```python
from build123d import *

# Parameters (mm, degrees)
SKETCH1_R           = 35.8013
SKETCH1_R_2         = 32.754
BOSS_EXTRUDE1_DEPTH = 15.875
CHAMFER1_SIZE       = 1.27


with BuildPart() as part:
    # Sketch1 → Boss-Extrude1 (new body, symmetric)
    with BuildSketch(Plane.XY):
        Circle(SKETCH1_R)
        Circle(SKETCH1_R_2, mode=Mode.SUBTRACT)
    extrude(amount=BOSS_EXTRUDE1_DEPTH, both=True)

    # Chamfer1
    chamfer1_edges = [part.edges().sort_by_distance(p)[0] for p in [
        (-32.754, 0, -15.875),
        (-32.754, 0, 15.875),
    ]]
    chamfer(chamfer1_edges, length=CHAMFER1_SIZE)

    # Sketch6 → Cut-Revolve2 (revolve, cut)
    with BuildSketch(Plane(origin=(0, 0, 0), x_dir=(1, 0, 0), z_dir=(0, 1, 0))):
        with BuildLine():
            Line((34.659, -8.597663689), (34.659, 8.597663689))
            ThreePointArc((34.659, 8.597663689), (34.949905783, 10.726866151), (35.8013, 12.7))
            Line((35.8013, 12.7), (35.8013, -12.7))
            ThreePointArc((35.8013, -12.7), (34.949905783, -10.726866151), (34.659, -8.597663689))
        make_face()
    revolve(axis=Axis((0, 0, -15.875), (0, 0, 1)), mode=Mode.SUBTRACT)


solid = part.part
```
Geometry: final body of the model. Coordinates: model frame, mm. Coordinates: 2 decimals unless noted, no trailing zeros. Order: outer loops, then holes, each group sorted by start corner. A loop starts at its lowest first (then second) coordinate and runs counter-clockwise, first axis right, second up. Notation, with made-up numbers: (7.5, 48) -> (47.5, 48) arc R13 ccw to (47.5, 61) -> close; hole circle Ø3 at (19, 83). An arc over 180 degrees is marked (long way). Answer in a Markdown table with one row per item.
Item 1: Section C-C on z = -2.5. Output: boundary loops of the cut face in (x, y).
Return value:
| item | result |
|---|---|
| outline | circle Ø69.32 at (0, 0); hole circle Ø65.51 at (0, 0) |
Item 2: Ray query, L1, parallel to Y at x = 0, z = -3.25; L2, parallel to X at y = 27, z = 2; L3, parallel to X at y = -28, z = -10. Return the intervals inside material, ascending.
Return value:
| item | result |
|---|---|
| L1 | y = -34.66 to -32.75, 32.75 to 34.66 |
| L2 | x = -21.73 to -18.54, 18.54 to 21.73 |
| L3 | x = -20.64 to -16.99, 16.99 to 20.64 |
Item 3: Draft query along Z for faces 1 (the cylindrical face through (15.99, -30.75, -0.12)), 2 (the flat face through (32, -13, -15.875)), 3 (the flat face through (32, -13, 15.875)), 4 (the cylindrical face through (-7.76, -34.95, 14.31)). Return one class per face: released by +Z, released by -Z, zero draft, split by the parting line, or undercut.
Return value:
| item | result |
|---|---|
| face 1 | undercut |
| face 2 | released by -Z |
| face 3 | released by +Z |
| face 4 | zero draft |
Item 4: Contact query for flat-ended pins moving along their axis: P1, Ø4, axis at y = -2, z = -7.5, coming from the -X side; P2, Ø6, axis at x = -18.5, z = 12.5, coming from the +Y side; P3, Ø12, axis at y = 16.5, z = 10, coming from the +X side; P4, Ø12, axis at x = -2.5, y = -21.5, coming from the -Z side. Output: stop coordinate, or through.
Return value:
| item | result |
|---|---|
| P1 | stops at x = -34.67 |
| P2 | stops at y = 32.27 |
| P3 | stops at x = 34.02 |
| P4 | passes through |
Item 5: Section A-A on x = 0. Output: boundary loops of the cut face in (y, z) (1 decimal), plus the area to 3 significant figures.
Return value:
| item | result |
|---|---|
| outline | (-35.8, -15.9) -> (-34, -15.9) -> (-32.8, -14.6) -> (-32.8, 14.6) -> (-34, 15.9) -> (-35.8, 15.9) -> (-35.8, 12.7) arc R7.9 cw to (-34.7, 8.6) -> (-34.7, -8.6) arc R7.9 cw to (-35.8, -12.7) -> close; (32.8, -14.6) -> (34, -15.9) -> (35.8, -15.9) -> (35.8, -12.7) arc R7.9 cw to (34.7, -8.6) -> (34.7, 8.6) arc R7.9 cw to (35.8, 12.7) -> (35.8, 15.9) -> (34, 15.9) -> (32.8, 14.6) -> close |
| area | 138 mm² |
